```python
from build123d import *


with BuildPart() as part:
    # Sketch1 → Revolve1 (revolve)
    with BuildSketch(Plane.XY):
        with BuildLine():
            Line((0, 8), (4, 8))
            Line((4, 8), (4, 12))
            Line((4, 12), (8, 16))
            Line((8, 16), (16.5, 16))
            Line((16.5, 16), (23, 22.5))
            Line((23, 22.5), (50, 22.5))
            ThreePointArc((50, 22.5), (52.121320344, 21.621320344), (53, 19.5))
            Line((53, 19.5), (53, 15))
            Line((53, 15), (25.772080403, 14.049180096))
            ThreePointArc((25.772080403, 14.049180096), (25.22452816, 13.805394131), (25, 13.249667434))
            Line((25, 13.249667434), (25, 5.1))
            Line((25, 5.1), (0, 5.1))
            Line((0, 5.1), (0, 8))
        make_face()
    revolve(axis=Axis((0, 0, 0), (1, 0, 0)))


solid = part.part
```
Check sheet for the modelled part. Datum: model origin and axes. Units: mm. A direction names the side the tool comes from. Coordinates: 2 decimals unless noted, no trailing zeros. Write each loop counter-clockwise with the first axis right and the second up, starting at its lowest first coordinate (ties: lowest second). Pieces come first, ordered by that corner, then holes. Notation, with made-up numbers: M -12,72 L 14,72 A14 ccw 14,99 Z; hole C 46.5,-23.75 d9. An arc over 180 degrees is marked long. Write item = value, one per line. Start each with the question number.
1. Sectioned sample at C-C (x = 24). Record the cut outline in (y, z), then the cut area to 3 significant figures.
2. Sectioned sample at D-D (x = 13.5). Record the cut outline in (y, z).
3. Mould release check, pull along Z, two halves, no side actions. Record for faces 1 (the cylindrical face through (12.3, 2.4, -4.5)), 2 (the flat face through (0, -5, -2)), 3 (the conical face through (16.91, 15.65, 4.93)): pulls with the +Z half, pulls with the -Z half, needs draft (parallel to the pull), parting line crosses it, or undercut.
4. Tool access check on faces 4 (the flat face through (25, 0, -6)), 5 (the cylindrical face through (2.03, -1.73, -7.81)), 6 (the flat face through (53, 10, -11.5)). Record the directions out of +Z, -Z, +X, -X, +Y, -Y that give a thin tool (end or side, any length) a straight path to the whole face; none if there is none.
5. Sectioned sample at A-A (z = 0). Record the cut outline in (x, y), then the cut area to 3 significant figures.
6. Thickness scan on probe 1 along Z at (x, y) = (12, 0); probe 2 along Z at (x, y) = (20, 0); probe 3 along X at (y, z) = (7.5, -8.5). Record the ranges inside material, lowest first.
7. Go/stop test with flat-tipped pins: pin 1 (6 mm diameter, centred on x = 38.5, y = -13.5, fed in from -Z); pin 2 (12 mm diameter, centred on x = 31.5, y = -14.5, fed in from +Z); pin 3 (2 mm diameter, centred on y = -6, z = -8, fed in from +X). Record where each tip stops, or that it passes through.
The answers:
q1.outline = C 0,0 d45; hole C 0,0 d10.2
q1.area = 1,510 mm²
q2.outline = C 0,0 d32; hole C 0,0 d10.2
q3.face_1 = undercut
q3.face_2 = needs draft
q3.face_3 = parting line crosses it
q4.face_4 = +X
q4.face_5 = -X
q4.face_6 = +Z, -Z, +X, +Y, -Y
q5.outline = M 0,-8 L 4,-8 L 4,-12 L 8,-16 L 16.5,-16 L 23,-22.5 L 50,-22.5 A3 ccw 53,-19.5 L 53,-15 L 25.77,-14.05 A0.8 cw 25,-13.25 L 25,-5.1 L 0,-5.1 Z; M 0,5.1 L 25,5.1 L 25,13.25 A0.8 cw 25.77,14.05 L 53,15 L 53,19.5 A3 ccw 50,22.5 L 23,22.5 L 16.5,16 L 8,16 L 4,12 L 4,8 L 0,8 Z
q5.area = 977 mm²
q6.probe_1 = -16 to -5.1, 5.1 to 16
q6.probe_2 = -19.5 to -5.1, 5.1 to 19.5
q6.probe_3 = 4 to 25
q7.pin_1 = -19.9
q7.pin_2 = 20.83
q7.pin_3 = 25
